Build history of the part. All positions in model axes, mm. Face numbers are marked on the shaded views. A direction names the side the tool comes from. Give positions to 0.01 mm unless a question says otherwise; leave off trailing zeros. Order: outer loops, then holes, each group sorted by start corner. A loop starts at its lowest first (then second) coordinate and runs counter-clockwise, first axis right, second up. Notation, with made-up numbers: M 17,41.25 L 70,41.25 A16 ccw 70,47.25 Z; hole C -13.5,85 d11. An arc over 180 degrees is marked long. One line per item, written item: value.
from build123d import *

# Parameters (mm, degrees)
SKETCH1_R           = 10.5
BOSS_EXTRUDE1_DEPTH = 15
SKETCH2_R           = 8
CUT_EXTRUDE1_DEPTH  = 7.5
SKETCH3_R           = 3
CUT_EXTRUDE2_DEPTH  = 7.5
CHAMFER1_SIZE       = 5


with BuildPart() as part:
    # Sketch1 → Boss-Extrude1 (new body)
    with BuildSketch(Plane(origin=(0, 0, 0), x_dir=(1, 0, 0), z_dir=(0, 1, 0))):
        with Locations(Location((0, 0, 0), (0, 0, 270))):
            Circle(SKETCH1_R)
    extrude(amount=BOSS_EXTRUDE1_DEPTH)

    # Sketch2 → Cut-Extrude1 (cut)
    with BuildSketch(Plane(origin=(0, 15, 0), x_dir=(1, 0, 0), z_dir=(0, 1, 0))):
        with Locations(Location((0, 0, 0), (0, 0, 270))):
            Circle(SKETCH2_R)
    extrude(amount=-CUT_EXTRUDE1_DEPTH, mode=Mode.SUBTRACT)

    # Sketch3 → Cut-Extrude2 (cut)
    with BuildSketch(Plane.XZ):
        with Locations(Location((0, 0, 0), (0, 0, 270))):
            Circle(SKETCH3_R)
    extrude(amount=-CUT_EXTRUDE2_DEPTH, mode=Mode.SUBTRACT)

    # Chamfer1
    chamfer1_edges = [part.edges().sort_by_distance(p)[0] for p in [
        (0, 0, -10.5),
    ]]
    chamfer(chamfer1_edges, length=CHAMFER1_SIZE)


solid = part.part
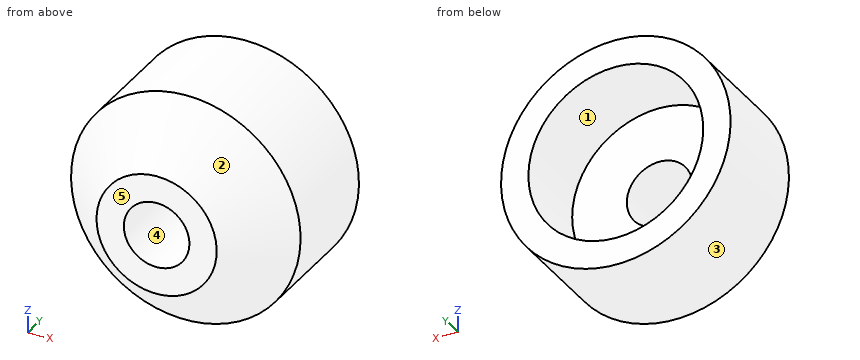
1) Saw through at D-D, the plane y = 5.75. Write the cut outline in (x, z).
Check values:
outline: C 0,0 d21; hole C 0,0 d6
2) Drill centre lines: probe 1 along X at (y, z) = (12, 0); probe 2 along X at (y, z) = (2.5, 0); probe 3 along Y at (x, z) = (2, -5). Where is each one in solid material? Low to high. Write a range as from..to.
Check values:
probe 1: -10.5..-8, 8..10.5
probe 2: -8..-3, 3..8
probe 3: 0..7.5
3) Tool access for the marked faces 1 and 2: list every direction of +Z, -Z, +X, -X, +Y, -Y with a clear straight run to the whole face (end or side of a thin tool).
Check values:
face 1: +Y
face 2: -Y
4) Saw through at C-C, the plane y = 14. Write the cut outline in (x, z), then the cut area to 3 significant figures.
Check values:
outline: C 0,0 d21; hole C 0,0 d16
area: 145 mm^2
5) Mould opens along X. For the marked faces 3, 4 and 5 say: released by +X, released by -X, zero draft, split by the parting line, or undercut.
Check values:
face 3: split by the parting line
face 4: undercut
face 5: zero draft
6) Saw through at A-A, the plane x = 0. Write the cut outline in (y, z), then the cut area to 3 significant figures.
Check values:
outline: M 0,-5.5 L 5,-10.5 L 15,-10.5 L 15,-8 L 7.5,-8 L 7.5,-3 L 0,-3 Z; M 0,3 L 7.5,3 L 7.5,8 L 15,8 L 15,10.5 L 5,10.5 L 0,5.5 Z
area: 125 mm^2
7) Pin check, flat tips, straight feed: pin 1 (1.5 mm diameter, centred on x = 8, z = 4, fed in from -Y); pin 2 (7 mm diameter, centred on x = 0, z = 0, fed in from +Y); pin 3 (3 mm diameter, centred on x = 5, y = 11.5, fed in from +Z). Stop position of each tip, or through.
Check values:
pin 1: y = 2.69
pin 2: y = 7.5
pin 3: z = 9.9
8) Saw through at B-B, the plane z = 0. Write the cut outline in (x, y), then the cut area to 3 significant figures.
Check values:
outline: M -10.5,5 L -5.5,0 L -3,0 L -3,7.5 L -8,7.5 L -8,15 L -10.5,15 Z; M 3,0 L 5.5,0 L 10.5,5 L 10.5,15 L 8,15 L 8,7.5 L 3,7.5 Z
area: 125 mm^2
